```python
from build123d import *

# Parameters (mm, degrees)
F0_R     = 84.1375
F1_DEPTH = 247.65
F2_R     = 31.75
F3_DEPTH = 5.08
F5_DEPTH = 25.4
F6_R     = 26.67
F7_DEPTH = 25.4


# Not quite as in the source:
# - a feature names something its author has since deleted; it is built from what else it names


with BuildPart() as f1:
    # F0 (on Front) → F1 (new body)
    with BuildSketch(Plane.XZ):
        Circle(F0_R)
    extrude(amount=F1_DEPTH)

    # F2 (on face) → F3 (join)
    with BuildSketch(Plane.XZ.offset(247.65)):
        Circle(F2_R)
    extrude(amount=F3_DEPTH)

    # F4 (on face) → F5 (cut)
    with BuildSketch(Plane.XZ.offset(247.65)):
        with BuildLine():
            ThreePointArc((-27.94, 33.02), (-29.4278975516, 36.6121024484), (-33.02, 38.1))
            ThreePointArc((-33.02, 38.1), (-36.6121024484, 36.6121024484), (-38.1, 33.02))
            ThreePointArc((-38.1, 33.02), (-33.02, 27.94), (-27.94, 33.02))
        make_face()
        with BuildLine():
            ThreePointArc((38.1, 33.02), (36.6121024484, 36.6121024484), (33.02, 38.1))
            ThreePointArc((33.02, 38.1), (29.4278975516, 29.4278975516), (38.1, 33.02))
        make_face()
        with BuildLine():
            ThreePointArc((33.02, -38.1), (36.6121024484, -36.6121024484), (38.1, -33.02))
            ThreePointArc((38.1, -33.02), (29.4278975516, -29.4278975516), (33.02, -38.1))
        make_face()
        with BuildLine():
            ThreePointArc((-27.94, -33.02), (-33.02, -27.94), (-38.1, -33.02))
            ThreePointArc((-38.1, -33.02), (-36.6121024484, -36.6121024484), (-33.02, -38.1))
            ThreePointArc((-33.02, -38.1), (-29.4278975516, -36.6121024484), (-27.94, -33.02))
        make_face()
    extrude(amount=-F5_DEPTH, mode=Mode.SUBTRACT)

    # F6 (on face) → F7 (cut)
    with BuildSketch(Plane.XZ.offset(252.73)):
        Circle(F6_R)
    extrude(amount=-F7_DEPTH, mode=Mode.SUBTRACT)


solid = f1.part
```
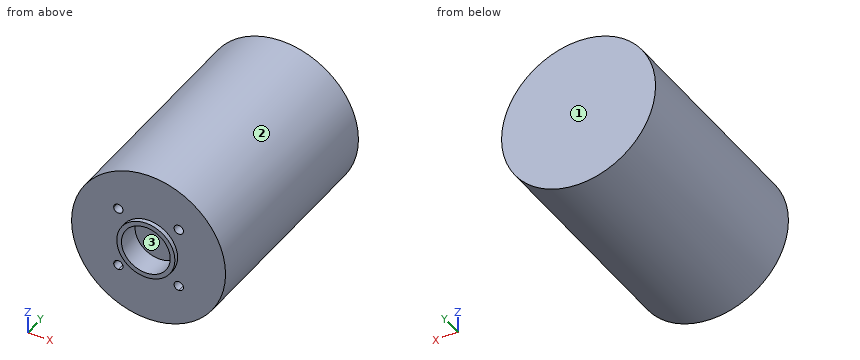
Read the model definition and answer for the solid it produces. Units are mm, in the model's axes. Face numbers are marked on the shaded views. Coordinates: 2 decimals unless noted, no trailing zeros. Write each loop counter-clockwise with the first axis right and the second up, starting at its lowest first coordinate (ties: lowest second). Pieces come first, ordered by that corner, then holes. Notation, with made-up numbers: (-5, -31.75) -> (43, -31.75) arc R27 ccw to (43, -2.75) -> close; hole circle Ø5 at (47.5, 54.25). An arc over 180 degrees is marked (long way). Answer as a JSON object with one key per item and string values.
Q1. The part is cut by section D-D on x = 59. Give the vertices of the cut face in (y, z), then the cut area to 3 significant figures.
The answers:
{"outline": "(-247.65, -59.98) -> (0, -59.98) -> (0, 59.98) -> (-247.65, 59.98) -> close", "area": "29,700 mm2"}
Q2. Consider line 1 (Z direction, x = 33.02, y = -241.75); line 2 (X direction, y = -232, z = 33); line 3 (Z direction, x = 0, y = -241.5). Determine where each line is inside the solid, lowest interval first. Write a range as [from, to].
The answers:
{"line 1": "z = [-77.39, -38.1], [-27.94, 27.94], [38.1, 77.39]", "line 2": "x = [-77.4, -38.1], [-27.94, 27.94], [38.1, 77.4]", "line 3": "z = [-84.14, -26.67], [26.67, 84.14]"}
Q3. The part is cut by section C-C on y = -199. Give the vertices of the cut face in (x, z) (1 decimal), then the cut area to 3 significant figures.
The answers:
{"outline": "circle Ø168.3 at (0, 0)", "area": "22,200 mm2"}
Q4. The part is cut by section A-A on z = 0. Give the vertices of the cut face in (x, y), then the cut area to 3 significant figures.
The answers:
{"outline": "(-84.14, -247.65) -> (-31.75, -247.65) -> (-31.75, -252.73) -> (-26.67, -252.73) -> (-26.67, -227.33) -> (26.67, -227.33) -> (26.67, -252.73) -> (31.75, -252.73) -> (31.75, -247.65) -> (84.14, -247.65) -> (84.14, 0) -> (-84.14, 0) -> close", "area": "40,600 mm2"}
Q5. Determine the mould class of the marked faces 1, 2 and 3 for opening direction Z: pulls with the +Z half, pulls with the -Z half, needs draft (parallel to the pull), parting line crosses it, or undercut.
The answers:
{"face 1": "needs draft", "face 2": "parting line crosses it", "face 3": "undercut"}
Q6. The part is cut by section B-B on x = 0. Give the vertices of the cut face in (y, z), then the cut area to 3 significant figures.
The answers:
{"outline": "(-252.73, -31.75) -> (-247.65, -31.75) -> (-247.65, -84.14) -> (0, -84.14) -> (0, 84.14) -> (-247.65, 84.14) -> (-247.65, 31.75) -> (-252.73, 31.75) -> (-252.73, 26.67) -> (-227.33, 26.67) -> (-227.33, -26.67) -> (-252.73, -26.67) -> close", "area": "40,600 mm2"}
Q7. Flat-ended cylindrical pins translate along their axes: pin 1 Ø10 at (y, z) = (-106, 7.5) entering from +X; pin 2 Ø10 at (x, z) = (-31, -67) entering from +Y; pin 3 Ø11 at (x, z) = (-34.5, 31.5) entering from -Y; pin 4 Ø4 at (y, z) = (-100, -58.5) entering from +X. Find the tip coordinate at first contact, or state that the pin passes through.
The answers:
{"pin 1": "stops at x = 84.1", "pin 2": "stops at y = 0", "pin 3": "stops at y = -247.65", "pin 4": "stops at x = 62.34"}
